```python
from build123d import *

# Parameters (mm, degrees)
BOSS_EXTRU_1_DEPTH      = 1
ESQUISSE2_W             = 13
ESQUISSE2_H             = 2
ENL_V_MAT_EXTRU_1_DEPTH = 1
CHANFREIN1_SIZE         = 2
ESQUISSE3_W             = 27.3
ESQUISSE3_H             = 19
BOSS_EXTRU_2_DEPTH      = 1
EPAISSIR1_START         = -6
EPAISSIR1_DEPTH         = 12


# Read off the part's stored shape, not the designer's step: Epaissir1
with BuildPart() as part:
    # Esquisse1 → Boss.-Extru.1 (new body)
    with BuildSketch(Plane.XY):
        Polygon((-11.65, -13.65), (11.65, -13.65), (13.65, -11.65), (13.65, 11.65), (11.65, 13.65), (-11.65, 13.65), (-13.65, 11.65), (-13.65, -11.65), align=None)
        with BuildLine():
            Line((-11, 12.7), (-9.7, 12.7))
            ThreePointArc((-9.7, 12.7), (-8.6, 11.6), (-9.7, 10.5))
            Line((-9.7, 10.5), (-11, 10.5))
            ThreePointArc((-11, 10.5), (-12.1, 11.6), (-11, 12.7))
        make_face(mode=Mode.SUBTRACT)
        with BuildLine():
            Line((11, 10.5), (9.7, 10.5))
            ThreePointArc((9.7, 10.5), (8.6, 11.6), (9.7, 12.7))
            Line((9.7, 12.7), (11, 12.7))
            ThreePointArc((11, 12.7), (12.1, 11.6), (11, 10.5))
        make_face(mode=Mode.SUBTRACT)
        with BuildLine():
            Line((-9.7, -12.7), (-11, -12.7))
            ThreePointArc((-11, -12.7), (-12.1, -11.6), (-11, -10.5))
            Line((-11, -10.5), (-9.7, -10.5))
            ThreePointArc((-9.7, -10.5), (-8.6, -11.6), (-9.7, -12.7))
        make_face(mode=Mode.SUBTRACT)
        with BuildLine():
            Line((11, -12.7), (9.7, -12.7))
            ThreePointArc((9.7, -12.7), (8.6, -11.6), (9.7, -10.5))
            Line((9.7, -10.5), (11, -10.5))
            ThreePointArc((11, -10.5), (12.1, -11.6), (11, -12.7))
        make_face(mode=Mode.SUBTRACT)
    extrude(amount=BOSS_EXTRU_1_DEPTH)

    # Esquisse2 → Enlèv. mat.-Extru.1 (cut)
    with BuildSketch(Plane.XY.offset(1)):
        with Locations((0, -12.65)):
            Rectangle(ESQUISSE2_W, ESQUISSE2_H)
    extrude(amount=-ENL_V_MAT_EXTRU_1_DEPTH, mode=Mode.SUBTRACT)

    # Chanfrein1
    chanfrein1_edges = [part.edges().sort_by_distance(p)[0] for p in [
        (6.5, -13.65, 0.5),
        (-6.5, -13.65, 0.5),
    ]]
    chamfer(chanfrein1_edges, length=CHANFREIN1_SIZE - 0.0001)  # a hair under: the kernel refuses the full size

    # Esquisse3 → Boss.-Extru.2 (add)
    with BuildSketch(Plane.XY.offset(1)):
        Rectangle(ESQUISSE3_W, ESQUISSE3_H)
    extrude(amount=BOSS_EXTRU_2_DEPTH)

    # Epaissir1 outline → Epaissir1 (add)
    with BuildSketch(Plane.YZ.offset(EPAISSIR1_START)):
        with BuildLine():
            add(Edge.make_bspline(
                [(-9.499999995, 1.979316014), (-9.705853917, 1.92496296), (-9.931420369, 1.860310756), (-10.169329786, 1.786375477), (-10.412025746, 1.704596537), (-10.652655847, 1.615090027), (-10.882677939, 1.520886463), (-11.096569941, 1.420298319), (-11.284403569, 1.317540699), (-11.441426278, 1.21133535), (-11.557190783, 1.104332165), (-11.626236767, 1.000000099)],
                knots=[0.002227245, 0.002227245, 0.002227245, 0.002227245, 0.002227245, 0.002227245, 0.002227245, 0.002227245, 0.002227245, 0.002227245, 0.002227245, 0.002227245, 0.990890106, 0.990890106, 0.990890106, 0.990890106, 0.990890106, 0.990890106, 0.990890106, 0.990890106, 0.990890106, 0.990890106, 0.990890106, 0.990890106], degree=11))
            Line((-9.499999995, 1.979316014), (-9.5, 2))
            add(Edge.make_bspline(
                [(-9.5, 2), (-10.263312196, 1.798883013), (-11.398783911, 1.403961588), (-11.65, 1)],
                knots=[0, 0, 0, 0, 1, 1, 1, 1], degree=3))
            Line((-11.65, 1), (-11.626236767, 1.000000099))
        make_face()
    extrude(amount=EPAISSIR1_DEPTH)


solid = part.part
```
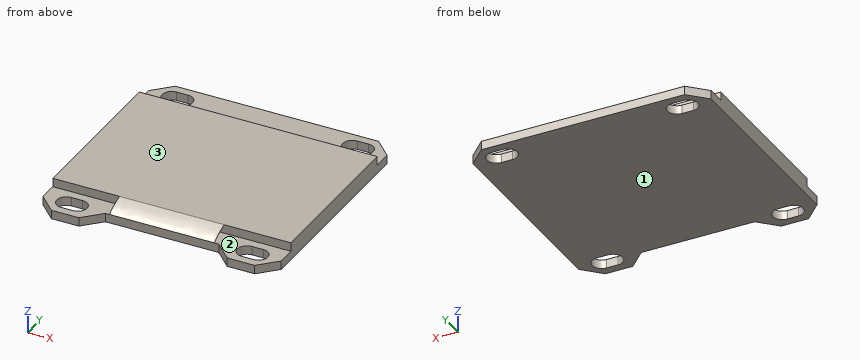
Design review of the part built by this model. Coordinates are the model's own, in mm. Face numbers are marked on the shaded views. Round coordinates to 2 decimals unless told otherwise and drop trailing zeros. Answer in a Markdown table with one row per item.
Q1. Clearance check with flat-ended pins moving along their axes: pin 1 Ø0.8 at (x, z) = (-4, 1.5) entering from -Y; pin 2 Ø1.2 at (x, y) = (6, 10.5) entering from +Z. State where each tip first meets the part, or that it passes through.
The answers:
| item | result |
|---|---|
| pin 1 | y = -11.57 |
| pin 2 | z = 1 |
Q2. Draft analysis for pull direction Z (two halves, no side actions). For the marked faces 1, 2 and 3, state which applies: +Z half, -Z half, draft (parallel to the pull), parting line (faces both ways), or undercut.
The answers:
| item | result |
|---|---|
| face 1 | -Z half |
| face 2 | undercut |
| face 3 | +Z half |
Q3. To check wall thickness, follow L1, parallel to Y at x = 10.5, z = 0.5; L2, parallel to Y at x = 9, z = 0.65; L3, parallel to Y at x = -9, z = 1.35. State the ranges of each line that lie inside material, in increasing order. Write a range as [from, to].
The answers:
| item | result |
|---|---|
| L1 | [-13.65, -12.7], [-10.5, 10.5], [12.7, 13.65] |
| L2 | [-13.65, -12.45], [-10.75, 10.75], [12.45, 13.65] |
| L3 | [-9.5, 9.5] |
Q4. Take a section at A-A, the plane z = 0.6. Count the separate pieces of the cut face and the enclosed holes in it, then the cut area to 3 significant figures.
The answers:
| item | result |
|---|---|
| separate pieces | 1 |
| enclosed holes | 4 |
| area | 681 mm² |
